Build history of the part. All positions in model axes, mm. A direction names the side the tool comes from. Round coordinates to 2 decimals unless told otherwise and drop trailing zeros. Loops run counter-clockwise (first coordinate to the right, second up) from the corner with the lowest first, then second, coordinate; pieces in that order, holes last. Notation, with made-up numbers: (72.25, 70) - (91.25, 70) arc R27 cw to (91.25, 107) - close; hole circle Ø3 at (-20, 44). An arc over 180 degrees is marked (long way). One line per question, with ' | ' between items. Start each with the question number.
from build123d import *

# Parameters (mm, degrees)
SKETCH_1_W          = 19.5
SKETCH_1_H          = 40
EXTRUDE_1_DEPTH     = 1.5
SKETCH_2_R          = 1.5
EXTRUDE_2_DEPTH     = 1.5
SKETCH_3_R          = 1
CUT_EXTRUDE_1_DEPTH = 1.5
FILLET_1_R          = 0.5
SKETCH_4_W          = 12
SKETCH_4_H          = 5
EXTRUDE_3_DEPTH     = 8


with BuildPart() as part:
    # ｽｹｯﾁ1 → ﾎﾞｽ - 押し出し1 (new body)
    with BuildSketch(Plane.XY):
        Rectangle(SKETCH_1_W, SKETCH_1_H)
    extrude(amount=EXTRUDE_1_DEPTH)

    # ｽｹｯﾁ2 → ﾎﾞｽ - 押し出し2 (add)
    with BuildSketch(Plane.XY.offset(1.5)):
        with Locations((9.75, 10)):
            Circle(SKETCH_2_R)
        with Locations((-9.75, 10)):
            Circle(SKETCH_2_R)
        with Locations((0, -20)):
            Circle(SKETCH_2_R)
    extrude(amount=-EXTRUDE_2_DEPTH)

    # ｽｹｯﾁ3 → ｶｯﾄ - 押し出し1 (cut)
    with BuildSketch(Plane.XY.offset(1.5)):
        with Locations((-9.75, 10)):
            Circle(SKETCH_3_R)
        with Locations((9.75, 10)):
            Circle(SKETCH_3_R)
        with Locations((0, -20)):
            Circle(SKETCH_3_R)
    extrude(amount=-CUT_EXTRUDE_1_DEPTH, mode=Mode.SUBTRACT)

    # ﾌｨﾚｯﾄ1
    fillet_1_edges = [part.edges().sort_by_distance(p)[0] for p in [
        (9.75, 8.5, 0.75),
        (9.75, 11.5, 0.75),
        (-9.75, 11.5, 0.75),
        (-9.75, 8.5, 0.75),
        (-1.5, -20, 0.75),
        (1.5, -20, 0.75),
    ]]
    fillet(fillet_1_edges, radius=FILLET_1_R)

    # ｽｹｯﾁ4 → ﾎﾞｽ - 押し出し3 (add)
    with BuildSketch(Plane.XY.offset(1.5)):
        with Locations((0, 16.5)):
            Rectangle(SKETCH_4_W, SKETCH_4_H)
    extrude(amount=EXTRUDE_3_DEPTH)


solid = part.part
1) Tool access for faces 1 (the flat face through (-6, 16, 5)), 2 (the flat face through (0, 19, 5)), 3 (the flat face through (-9.75, -6, 1)), 4 (the flat face through (0, 14, 5)), 5 (the flat face through (9.75, 16, 1)): list every direction of +Z, -Z, +X, -X, +Y, -Y with a clear straight run to the whole face (end or side of a thin tool).
2) Saw through at A-A on y = 10. Write the cut outline in (x, z).
3) Saw through at C-C on z = 8.5. Write the cut outline in (x, y), and give its area (3 significant figures).
4) Saw through at D-D on x = -5. Write the cut outline in (y, z), and give its area (3 significant figures).
5) Wall check: line 1 (Y direction, x = 0, z = 1.1); line 2 (Z direction, x = 9, y = 6.5); line 3 (Y direction, x = -1, z = 6.25). Give the ranges that are in metal, low to high. Write a range as [from, to].
6) Two-plate mould, pull along Y, no slides. Class faces 6 (the flat face through (0, 0, 0)), 7 (the cylindrical face through (11.25, 9.97, 0.76)), 8 (the cylindrical face through (0, -21, 1)): +Y half, -Y half, draft (parallel to the pull), parting line (faces both ways), or undercut.
7) Drop flat-ended pins along their axis: pin 1 (0.8 mm diameter, centred on y = 15.5, z = 0.5, fed in from +X); pin 2 (2.5 mm diameter, centred on x = -1, z = 5.5, fed in from -Y); pin 3 (1.2 mm diameter, centred on x = 4, z = 1, fed in from -Y). Give the stop position or say it passes through.
8) Saw through at B-B on x = 0. Write the cut outline in (y, z), and give its area (4 significant figures).
Answer key:
1) face 1: +Z, -X, +Y, -Y | face 2: +Z, +X, -X, +Y | face 3: +Z, -Z, -X, -Y | face 4: +Z, +X, -X, -Y | face 5: +Z, -Z, +X, +Y
2) outline: (-11.25, 0) - (-10.75, 0) - (-10.75, 1.5) - (-11.25, 1.5) - close; (-8.75, 0) - (8.75, 0) - (8.75, 1.5) - (-8.75, 1.5) - close; (10.75, 0) - (11.25, 0) - (11.25, 1.5) - (10.75, 1.5) - close
3) outline: (-6, 14) - (6, 14) - (6, 19) - (-6, 19) - close | area: 60.0 mm²
4) outline: (-20, 0) - (20, 0) - (20, 1.5) - (19, 1.5) - (19, 9.5) - (14, 9.5) - (14, 1.5) - (-20, 1.5) - close | area: 100 mm²
5) line 1: [-21.5, -21], [-19, 20] | line 2: [0, 1.5] | line 3: [14, 19]
6) face 6: draft | face 7: parting line | face 8: undercut
7) pin 1: x = 9.75 | pin 2: y = 14 | pin 3: y = -20
8) outline: (-21.5, 0) - (-21, 0) - (-21, 1.5) - (-21.5, 1.5) - close; (-19, 0) - (20, 0) - (20, 1.5) - (19, 1.5) - (19, 9.5) - (14, 9.5) - (14, 1.5) - (-19, 1.5) - close | area: 99.25 mm²
